Design review of the part built by this model. Coordinates are the model's own, in mm. A direction names the side the tool comes from. Round coordinates to 2 decimals unless told otherwise and drop trailing zeros. Order: outer loops, then holes, each group sorted by start corner. A loop starts at its lowest first (then second) coordinate and runs counter-clockwise, first axis right, second up. Notation, with made-up numbers: M -26.5,-16 L 12.5,-16 A13 ccw 12.5,-3 Z; hole C 52.25,-7 d5. An arc over 180 degrees is marked long. Write item = value, one per line. Start each with the question number.
```python
from build123d import *

# Parameters (mm, degrees)
F0_W = 6
F0_H = 10
F2_W = 3
F2_H = 3


# Not quite as in the source:
# - ends of sketch curves that miss each other by under 0.0002 mm in the source are joined


with BuildPart() as f3:
    # F0 (on Front) → F3 section 0
    with BuildSketch(Plane.XZ):
        Rectangle(F0_W, F0_H)
    # F2 (on offset) → F3 section 1
    with BuildSketch(Plane.XZ.offset(-65)):
        Rectangle(F2_W, F2_H)
    loft()


with BuildPart() as f5:
    # F4 (on Right) → F5 (revolve)
    with BuildSketch(Plane.YZ):
        with BuildLine():
            Line((10, 15), (0, 5))
            Line((0, 5), (0, 0))
            Line((0, 0), (106, 0))
            ThreePointArc((106, 0), (100.5324895422, 12.0443623345), (87.8666669945, 15.8571400412))
            Line((87.8666669945, 15.8571400412), (56.800088, 10.359742))
            ThreePointArc((56.800088, 10.359742), (35.7475326189, 9.4526994667), (15.1884568347, 14.0740865517))
            ThreePointArc((15.1884568347, 14.0740865517), (12.6352134757, 14.7667074847), (10, 15))
        make_face()
    revolve(axis=Axis((0, 53, 0), (0, 1, 0)))

    # F6: cut F3
    add(f3.part, mode=Mode.SUBTRACT)


solid = f5.part
```
(1) Consider section A-A, the plane y = 72. Write out the cut boundary in (x, z).
(2) Draft analysis for pull direction Y (two halves, no side actions). For faces 1 (the face through (-3.3, 0.5, -4.4)), 2 (the face through (3.742, 68.664, 11.884)), state which applies: pulls with the +Y half, pulls with the -Y half, needs draft (parallel to the pull), parting line crosses it, or undercut.
(3) Insertion check: pin 1 (1 mm diameter, centred on x = -6, z = 8, fed in from -Y); pin 2 (1.5 mm diameter, centred on x = 0, z = 0, fed in from -Y); pin 3 (3 mm diameter, centred on x = 10.5, z = 8.5, fed in from -Y); pin 4 (2 mm diameter, centred on x = -4, z = 0, fed in from -Y). Each pin has a flat end and moves straight along its axis. Give the tip position at first contact, or say it passes through.
(4) Consider section B-B, the plane y = 97. Write out the cut boundary in (x, z), then the cut area to 3 significant figures.
(5) For faces 3 (the face through (4, 0, 0)), 4 (the face through (0, 65, 0)), list the 3-axis set-ups (+Z, -Z, +X, -X, +Y, -Y) from which the entire face can be reached by the end or side of a thin tool; tool diameter is ignored.
(6) For line 1 along X through (y, z) = (15.5, 0); line 2 along X through (y, z) = (72.5, 1.5); line 3 along X through (y, z) = (72.5, -6), list the stretches that pass through material, from the lowest coordinate up. Write a range as [from, to].
Completed:
q1.outline = C 0,0 d26.1
q2.face_1 = pulls with the -Y half
q2.face_2 = undercut
q3.pin_1 = 4.5
q3.pin_2 = 65
q3.pin_3 = 7.01
q3.pin_4 = 0
q4.outline = C 0,0 d28.77
q4.area = 650 mm2
q5.face_3 = +Z, -Z, +X, -X, -Y
q5.face_4 = -Y
q6.line_1 = [-13.96, -2.64], [2.64, 13.96]
q6.line_2 = [-13.05, 13.05]
q6.line_3 = [-11.69, 11.69]
